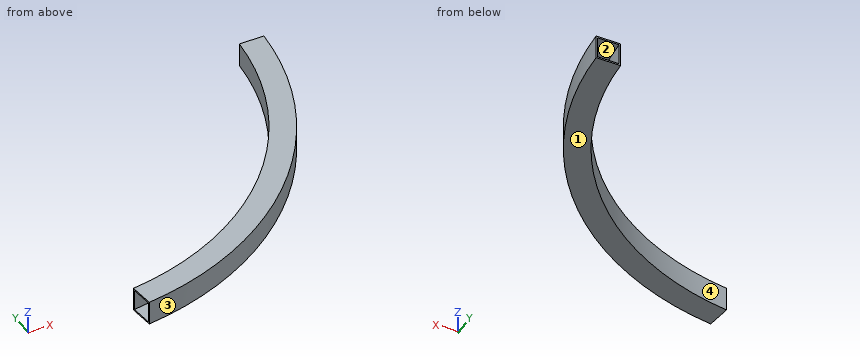
Autodesk Inventor part; units mm, degrees
ref_plane "YZ Plane" through (0, 0, 0) normal (1, 0, 0) x (0, 1, 0)
ref_plane "XZ Plane" through (0, 0, 0) normal (0, 1, 0) x (-1, 0, 0)
ref_plane "XY Plane" through (0, 0, 0) normal (0, 0, 1) x (1, 0, 0)
sketch "Sketch1" plane through (0, 0, 0) normal (0, 0, 1) x (1, 0, 0)
  arc A0 (38.1676, -289.5957) -> (291.8238, -12.7) centre (0, 0) ccw
  arc A1 (41.4865, -314.7779) -> (317.2459, -12.7) centre (0, 0) ccw
  line L0 (38.1676, -289.5957) -> (41.4865, -314.7779)
  line L1 (291.8238, -12.7) -> (317.2459, -12.7)
  line L2 (0, 0) -> (38.1676, -289.5957) construction
  line L3 (0, -292.1) -> (0, 0) construction
  line L4 (291.8238, -12.7) -> (0, 0) construction
  line L5 (291.8238, 0) -> (317.2459, 0) construction
  line L6 (317.2459, 0) -> (317.2459, -12.7) construction
  line L7 (317.2459, -12.7) -> (291.8238, -12.7) construction
  line L8 (291.8238, -12.7) -> (291.8238, 0) construction
  line L9 (0, 0) -> (359.7285, 0) construction
  dimension "d0" = 292.1
  dimension "d1" = 25.4
  dimension "d9" = 12.7
  dimension "d10" = 80
extrude "Extrusion1" add sketch "Sketch1" along normal blind 25.4
shell "Shell1" thickness 1.5875 removed faces 2 at (300.2978, -12.7, 8.4667) at (40.3802, -306.3838, 8.4667)
properties part number "Shooter_Frame_RearGuide" material "Aluminum-6061"
Geometry check sheet. Reference: the model listing, model coordinates, mm. Face numbers are marked on the shaded views. Give positions to 0.01 mm unless a question says otherwise; leave off trailing zeros. Write each loop counter-clockwise with the first axis right and the second up, starting at its lowest first coordinate (ties: lowest second). Pieces come first, ordered by that corner, then holes.
1) Cross-section at A-A (z = 6). Record the boundary of the cut face in (x, y), plus the area to 3 significant figures.
Values follow:
outline: (38.17, -289.6) - (38.38, -291.17) arc R293.69 ccw to (293.41, -12.7) - (291.82, -12.7) arc R292.1 cw to start; (41.28, -313.2) - (41.49, -314.78) arc R317.5 ccw to (317.25, -12.7) - (315.66, -12.7) arc R315.91 cw to start
area: 1,350 mm2
2) Thickness scan on line 1 (Y direction, x = 179.5, z = 6); line 2 (Y direction, x = 211, z = 21); line 3 (X direction, y = -115, z = 3.5). Record the ranges inside material, lowest first.
Values follow:
line 1: y = -261.89 to -259.96, -232.45 to -230.44
line 2: y = -237.25 to -235.12, -204.28 to -201.99
line 3: x = 268.51 to 270.24, 294.24 to 295.94
3) Release check for a two-part mould opening along X. For the marked faces 1, 2, 3 and 4 record: released by +X, released by -X, zero draft, split by the parting line, or undercut.
Values follow:
face 1: zero draft
face 2: undercut
face 3: released by +X
face 4: released by -X
4) Go/stop test with flat-tipped pins: pin 1 Ø1.5 at (x, z) = (95, 16.5) entering from +Y; pin 2 Ø2 at (x, z) = (138.5, 13.5) entering from +Y; pin 3 Ø5 at (x, z) = (114.5, 8.5) entering from -Y. Record where each tip stops, or that it passes through.
Values follow:
pin 1: stops at y = -275.96
pin 2: stops at y = -256.64
pin 3: stops at y = -297.09
5) Cross-section at B-B (x = 97.5). Record the boundary of the cut face in (y, z), plus the area to 3 significant figures.
Values follow:
outline: (-302.16, 0) - (-275.35, 0) - (-275.35, 25.4) - (-302.16, 25.4) - close; hole (-300.49, 1.59) - (-277.03, 1.59) - (-277.03, 23.81) - (-300.49, 23.81) - close
area: 160 mm2
6) Cross-section at C-C (y = -151.5). Record the boundary of the cut face in (x, z), plus the area to 3 significant figures.
Values follow:
outline: (249.74, 0) - (279.02, 0) - (279.02, 25.4) - (249.74, 25.4) - close; hole (251.6, 1.59) - (277.22, 1.59) - (277.22, 23.81) - (251.6, 23.81) - close
area: 174 mm2
